```python
from build123d import *

# Parameters (mm, degrees)
F0_W     = 100
F0_H     = 60
F1_DEPTH = 8
F2_R     = 3.99999


# Not quite as in the source:
# - a fillet or chamfer is up to 0.001 mm smaller than in the source, because OpenCascade refuses the exact size


with BuildPart() as f1:
    # F0 (on Top) → F1 (new body)
    with BuildSketch(Plane.XY):
        Rectangle(F0_W, F0_H)
    extrude(amount=F1_DEPTH)

    # F2 (radius 4 in the source; OpenCascade refuses exactly that, so slightly less here)
    f2_edges = [f1.edges().sort_by_distance(p)[0] for p in [
        (0, -30, 8),
        (0, -30, 0),
        (50, 0, 8),
        (50, 0, 0),
        (0, 30, 8),
        (0, 30, 0),
    ]]
    fillet(f2_edges, radius=F2_R)


solid = f1.part
```
For this review, take the finished solid that the model builds, in its own axes (mm). Round coordinates to 2 decimals unless told otherwise and drop trailing zeros. Loops run counter-clockwise (first coordinate to the right, second up) from the corner with the lowest first, then second, coordinate; pieces in that order, holes last.
Q1. To check wall thickness, follow line 1 along Y through (x, z) = (46.5, 5.75); line 2 along X through (y, z) = (-14.5, 3.5); line 3 along Y through (x, z) = (38.5, 3.5). State the ranges of each line that lie inside material, in increasing order.
Result sheet:
line 1: y = -29.6 to 29.6
line 2: x = -50 to 49.97
line 3: y = -29.97 to 29.97
Q2. Add section B-B on z = 5.75. Write out the cut boundary in (x, y), plus the area to 3 significant figures.
Result sheet:
outline: (-50, -29.6) - (49.6, -29.6) - (49.6, 29.6) - (-50, 29.6) - close
area: 5,900 mm2
Q3. Add section C-C on z = 1.25. Write out the cut boundary in (x, y), plus the area to 3 significant figures.
Result sheet:
outline: (-50, -28.9) - (48.9, -28.9) - (48.9, 28.9) - (-50, 28.9) - close
area: 5,720 mm2
Q4. Insertion check: pin 1 Ø1 at (y, z) = (13.5, 3) entering from +X. The pin has a flat end and moves straight along its axis. Give the tip position at first contact, or say it passes through.
Result sheet:
pin 1: stops at x = 49.97
